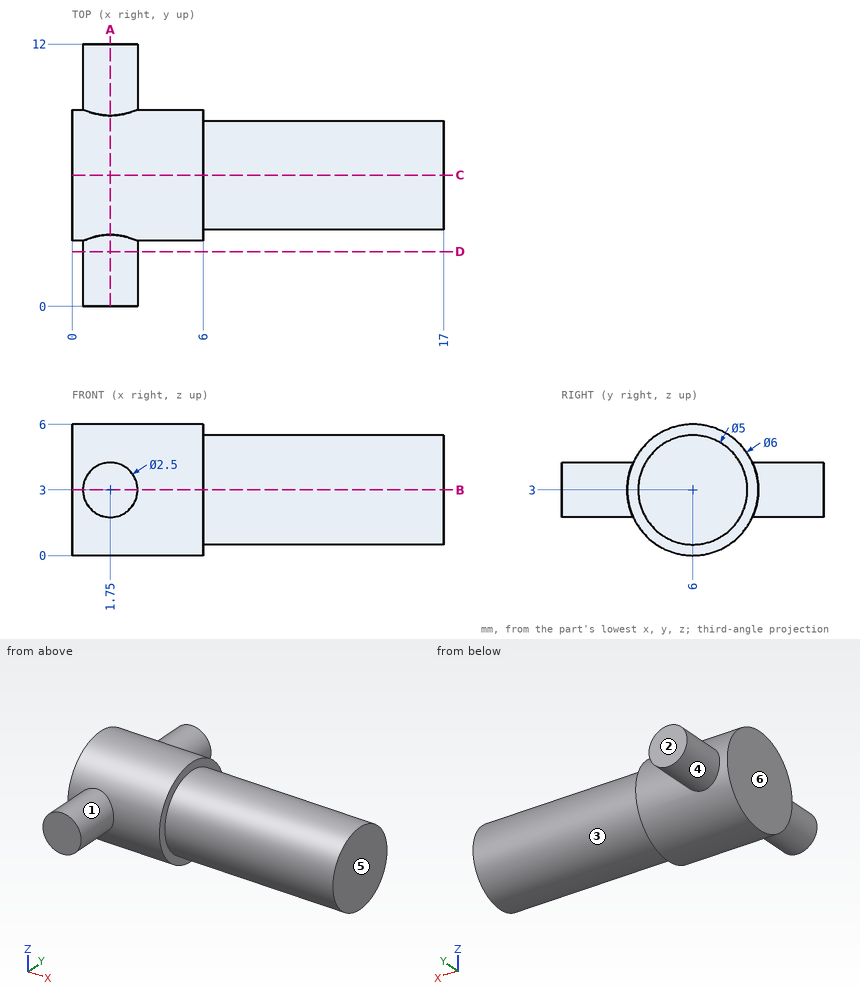
Print and shaded views of the part. All mm, measured from the part's lowest x, y and z. A direction names the side the tool comes from. Coordinates: 2 decimals unless noted, no trailing zeros. Order: outer loops, then holes, each group sorted by start corner. A loop starts at its lowest first (then second) coordinate and runs counter-clockwise, first axis right, second up. Notation, with made-up numbers: (-4.75, 51.5) -> (38.25, 51.5) arc R30 cw to (38.25, 77.5) -> close; hole circle Ø10 at (33.5, -31.75). An arc over 180 degrees is marked (long way). Use one line per item in the form item = value. Start each with the question number.
1) Drop flat-ended pins along their axis: pin 1 (3 mm diameter, centred on y = 10, z = 1.5, fed in from +X); pin 2 (1.5 mm diameter, centred on x = 13, y = 6, fed in from +Z). Give the stop position or say it passes through.
2) Band-saw the part on D-D on y = 2.5. Give the cut face in (x, z).
3) Band-saw the part on C-C on y = 6. Give the cut face in (x, z).
4) Band-saw the part on B-B on z = 3. Give the cut face in (x, y), then the cut area to 3 significant figures.
5) Drill centre lines: L1, parallel to X at y = 7, z = 5.75; L2, parallel to Y at x = 10, z = 2; L3, parallel to Y at x = 14, z = 4.75. Where is each one in solid material? Low to high. Write a range as [from, to].
6) Band-saw the part on A-A on x = 1.75. Give the cut face in (y, z).
7) Pull direction X, two halves, no side cores. Call the marked faces 3, 4, 5 and 6: +X half, -X half, draft (parallel to the pull), parting line (faces both ways), or undercut.
8) Tool access for the marked faces 1 and 2: list every direction of +Z, -Z, +X, -X, +Y, -Y with a clear straight run to the whole face (end or side of a thin tool).
Entries:
q1.pin_1 = 6
q1.pin_2 = 5.5
q2.outline = circle Ø2.5 at (1.75, 3)
q3.outline = (0, 0) -> (6, 0) -> (6, 0.5) -> (17, 0.5) -> (17, 5.5) -> (6, 5.5) -> (6, 6) -> (0, 6) -> close
q4.outline = (0, 3) -> (0.5, 3) -> (0.5, 0) -> (3, 0) -> (3, 3) -> (6, 3) -> (6, 3.5) -> (17, 3.5) -> (17, 8.5) -> (6, 8.5) -> (6, 9) -> (3, 9) -> (3, 12) -> (0.5, 12) -> (0.5, 9) -> (0, 9) -> close
q4.area = 106 mm2
q5.L1 = [0, 6]
q5.L2 = [3.71, 8.29]
q5.L3 = [4.21, 7.79]
q6.outline = (0, 1.75) -> (3.27, 1.75) arc R3 ccw to (8.73, 1.75) -> (12, 1.75) -> (12, 4.25) -> (8.73, 4.25) arc R3 ccw to (3.27, 4.25) -> (0, 4.25) -> close
q7.face_3 = draft
q7.face_4 = parting line
q7.face_5 = +X half
q7.face_6 = -X half
q8.face_1 = -Y
q8.face_2 = +Z, -Z, +X, -X, +Y
